Input: part model. Units: mm. Frame: model coordinates. Face numbers are marked on the shaded views. A direction names the side the tool comes from. Give positions to 0.01 mm unless a question says otherwise; leave off trailing zeros. Order: outer loops, then holes, each group sorted by start corner. A loop starts at its lowest first (then second) coordinate and runs counter-clockwise, first axis right, second up. Notation, with made-up numbers: (-13, 89.25) - (3, 89.25) arc R20 cw to (3, 96.25) - close; hole circle Ø8 at (81, -10.75). An arc over 180 degrees is marked (long way). Use a Markdown table: item, result.
from build123d import *

# Parameters (mm, degrees)
ESQUISSE2_W              = 30
ESQUISSE2_H              = 30
BOSS_EXTRU_1_DEPTH       = 5
ESQUISSE16_R             = 2.5
BOSS_EXTRU_7_DEPTH       = 6
CONG_3_R                 = 1
ESQUISSE18_R             = 2.5
BOSS_EXTRU_9_DEPTH       = 6
CONG_5_R                 = 1
ESQUISSE8_R              = 12.5
ENL_V_MAT_EXTRU_1_DEPTH  = 2
ESQUISSE19_R             = 7.5
BOSS_EXTRU_10_DEPTH      = 2
ESQUISSE33_R             = 4
ENL_V_MAT_EXTRU_3_DEPTH  = 6
ESQUISSE35_R             = 2.5
BOSS_EXTRU_26_DEPTH      = 6
CONG_6_R                 = 1
BOSS_EXTRU_27_DEPTH      = 2
BOSS_EXTRU_27_DEPTH_BACK = 5.5


with BuildPart() as part:
    # Esquisse2 → Boss.-Extru.1 (new body)
    with BuildSketch(Plane.XY):
        Rectangle(ESQUISSE2_W, ESQUISSE2_H)
    extrude(amount=BOSS_EXTRU_1_DEPTH)

    # Esquisse16 → Boss.-Extru.7 (add)
    with BuildSketch(Plane.ZY.offset(15)):
        with Locations((2.5, 7)):
            Circle(ESQUISSE16_R)
        with Locations((2.5, -7)):
            Circle(ESQUISSE16_R)
    extrude(amount=BOSS_EXTRU_7_DEPTH)

    # Congé3
    cong_3_edges = [part.edges().sort_by_distance(p)[0] for p in [
        (-21, 7, 0),
        (-21, -7, 0),
    ]]
    fillet(cong_3_edges, radius=CONG_3_R)

    # Esquisse18 → Boss.-Extru.9 (add)
    with BuildSketch(Plane(origin=(15, 0, 0), x_dir=(0, 0, -1), z_dir=(1, 0, 0))):
        with Locations((-2.5, 7)):
            Circle(ESQUISSE18_R)
    extrude(amount=BOSS_EXTRU_9_DEPTH)

    # Congé5
    cong_5_edges = [part.edges().sort_by_distance(p)[0] for p in [
        (21, 7, 5),
    ]]
    fillet(cong_5_edges, radius=CONG_5_R)

    # Esquisse8 → Enlèv. mat.-Extru.1 (cut)
    with BuildSketch(Plane.XY.offset(5)):
        Circle(ESQUISSE8_R)
    extrude(amount=-ENL_V_MAT_EXTRU_1_DEPTH, mode=Mode.SUBTRACT)

    # Esquisse19 → Boss.-Extru.10 (add)
    with BuildSketch(Plane.XY.offset(3)):
        Circle(ESQUISSE19_R)
    extrude(amount=BOSS_EXTRU_10_DEPTH)

    # Esquisse33 → Enlèv. mat.-Extru.3 (cut, through all)
    with BuildSketch(Plane.XY.offset(5)):
        Circle(ESQUISSE33_R)
    extrude(amount=-ENL_V_MAT_EXTRU_3_DEPTH, mode=Mode.SUBTRACT)

    # Esquisse35 → Boss.-Extru.26 (add)
    with BuildSketch(Plane(origin=(0, 15, 0), x_dir=(1, 0, 0), z_dir=(0, 1, 0))):
        with Locations((7, -2.5)):
            Circle(ESQUISSE35_R)
    extrude(amount=BOSS_EXTRU_26_DEPTH)

    # Congé6
    cong_6_edges = [part.edges().sort_by_distance(p)[0] for p in [
        (4.5, 21, 2.5),
    ]]
    fillet(cong_6_edges, radius=CONG_6_R)

    # Esquisse31 → Boss.-Extru.27 (add, two sides)
    with BuildSketch(Plane.XY.offset(3)) as boss_extru_27_sk:
        Polygon((-9.899494937, 7.778174593), (-7.778174593, 9.899494937), (-3.545672625, 5.666992969), (-5.666992969, 3.545672625), align=None)
    extrude(amount=BOSS_EXTRU_27_DEPTH)
    extrude(boss_extru_27_sk.sketch, amount=-BOSS_EXTRU_27_DEPTH_BACK)


solid = part.part
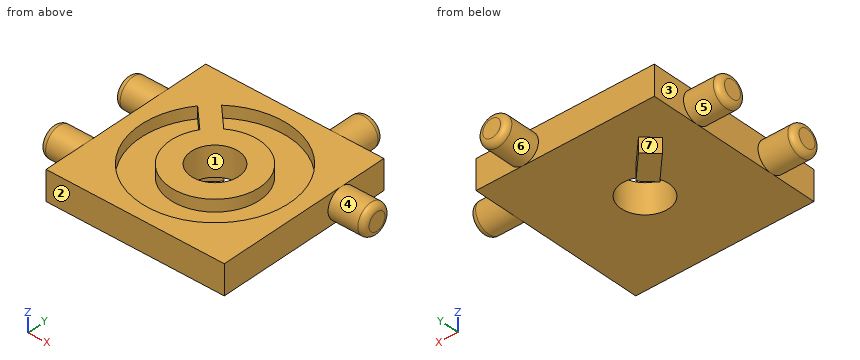
1. Set-up query: the marked faces 4, 5, 6 and 7. Return all of +Z, -Z, +X, -X, +Y, -Y with unobstructed straight access to the full face (end or side cutting, diameter ignored); none if empty.
Response:
| item | result |
|---|---|
| face 4 | +X |
| face 5 | -X |
| face 6 | +Y |
| face 7 | -Z, -X, +Y |
2. Material intervals for line 1 along Y through (x, z) = (0, 3.65); line 2 along Y through (x, z) = (3, 4), sorted ascending.
Response:
| item | result |
|---|---|
| line 1 | y = -15 to -12.5, -7.5 to -4, 4 to 7.5, 12.5 to 15 |
| line 2 | y = -15 to -12.13, -6.87 to -2.65, 2.65 to 6.87, 12.13 to 15 |
3. Section query A-A (y = 0). Return loops of the section in (x, z), then the cut area to 3 significant figures.
Response:
| item | result |
|---|---|
| outline | (-15, 0) - (-4, 0) - (-4, 5) - (-7.5, 5) - (-7.5, 3) - (-12.5, 3) - (-12.5, 5) - (-15, 5) - close; (4, 0) - (15, 0) - (15, 5) - (12.5, 5) - (12.5, 3) - (7.5, 3) - (7.5, 5) - (4, 5) - close |
| area | 90.0 mm^2 |
4. Section query D-D (x = 10). Return loops of the section in (y, z), then the cut area to 3 significant figures.
Response:
| item | result |
|---|---|
| outline | (-15, 0) - (15, 0) - (15, 5) - (7.5, 5) - (7.5, 3) - (-7.5, 3) - (-7.5, 5) - (-15, 5) - close |
| area | 120 mm^2 |
5. Mould query, pull axis Y, two halves, no side actions, for the marked faces 1, 2 and 3. Classes: pulls with the +Y half, pulls with the -Y half, needs draft (parallel to the pull), parting line crosses it, or undercut.
Response:
| item | result |
|---|---|
| face 1 | undercut |
| face 2 | pulls with the -Y half |
| face 3 | needs draft |
6. Pin query (flat end, axial travel): pin 1 (1 mm diameter, centred on y = -9.5, z = 2.5, fed in from +X); pin 2 (2.5 mm diameter, centred on x = 12, z = 3.5, fed in from +Y); pin 3 (1.5 mm diameter, centred on y = 0.5, z = 2.5, fed in from -X); pin 4 (20 mm diameter, centred on x = 0, y = -2.5, fed in from +Z). Return the tip coordinate at first contact, or that it passes through.
Response:
| item | result |
|---|---|
| pin 1 | stops at x = 15 |
| pin 2 | stops at y = 15 |
| pin 3 | stops at x = -15 |
| pin 4 | stops at z = 5 |
